Read the model definition and answer for the solid it produces. Units are mm, in the model's axes. Give positions to 0.01 mm unless a question says otherwise; leave off trailing zeros. Order: outer loops, then holes, each group sorted by start corner. A loop starts at its lowest first (then second) coordinate and runs counter-clockwise, first axis right, second up.
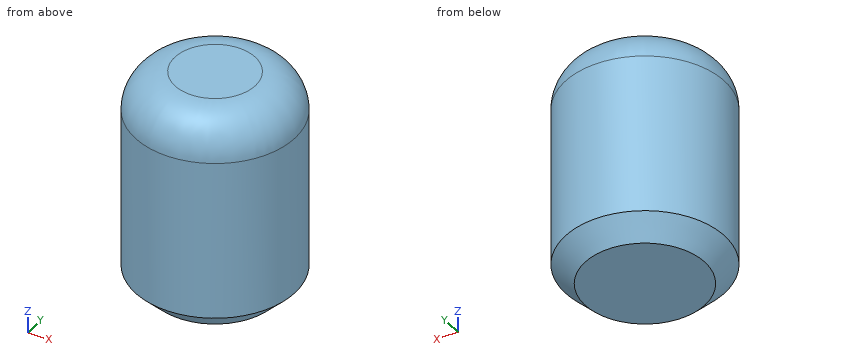
```python
from build123d import *

# Parameters (mm, degrees)
F0_R     = 20.1519646926
F1_DEPTH = 25.4
F2_DEPTH = 30
F3_R     = 10
F4_SIZE  = 5


with BuildPart() as f1:
    # F0 (on Top) → F1 (new body)
    with BuildSketch(Plane.XY):
        Circle(F0_R)
    extrude(amount=F1_DEPTH)

    # F2 (add): a face of the model
    f2_faces = [f1.faces().sort_by_distance(p)[0] for p in [
        (0, 0, 25.4),
    ]]
    extrude(f2_faces, amount=F2_DEPTH)

    # F3
    f3_edges = [f1.edges().sort_by_distance(p)[0] for p in [
        (-20.151965, 0, 55.4),
    ]]
    fillet(f3_edges, radius=F3_R)

    # F4
    f4_edges = [f1.edges().sort_by_distance(p)[0] for p in [
        (-20.151965, 0, 0),
    ]]
    chamfer(f4_edges, length=F4_SIZE)


solid = f1.part
```
1) Given pin 1 (6 mm diameter, centred on y = 12.5, z = 19.5, fed in from +X); pin 2 (10 mm diameter, centred on x = 11.5, z = 16, fed in from -Y); pin 3 (1 mm diameter, centred on x = 5, y = 10, fed in from +Z), each flat-ended and moving along its own axis, determine where each tip first touches the part or whether it passes through.
Final values:
pin 1: stops at x = 17.77
pin 2: stops at y = -19.07
pin 3: stops at z = 55.39
2) The part is cut by section C-C on z = 17.5. Determine the outline of the cut face in (x, y).
Final values:
outline: circle Ø40.3 at (0, 0)
3) Consider L1, parallel to Y at x = 0.5, z = 19.5; L2, parallel to X at y = -3.5, z = 4.5; L3, parallel to X at y = -4.5, z = 49. Determine where each line is inside the solid, lowest interval first.
Final values:
L1: y = -20.15 to 20.15
L2: x = -19.34 to 19.34
L3: x = -18.95 to 18.95
4) The part is cut by section A-A on y = 0. Determine the outline of the cut face in (x, z), and give its area (3 significant figures).
Final values:
outline: (-20.15, 5) - (-15.15, 0) - (15.15, 0) - (20.15, 5) - (20.15, 45.4) arc R10 ccw to (10.15, 55.4) - (-10.15, 55.4) arc R10 ccw to (-20.15, 45.4) - close
area: 2,160 mm2
